Part model, mm, in its own coordinate system. Round coordinates to 2 decimals unless told otherwise and drop trailing zeros. Write each loop counter-clockwise with the first axis right and the second up, starting at its lowest first coordinate (ties: lowest second). Pieces come first, ordered by that corner, then holes.
```python
from build123d import *

# Parameters (mm, degrees)
ESQUISSE1_W             = 310
ESQUISSE1_H             = 380
BOSS_EXTRU_1_DEPTH      = 4
CONG_1_R                = 5
ESQUISSE3_R             = 10.5
ESQUISSE3_R_2           = 11
ESQUISSE3_R_3           = 2.5
ENL_V_MAT_EXTRU_1_DEPTH = 10


with BuildPart() as part:
    # Esquisse1 → Boss.-Extru.1 (new body)
    with BuildSketch(Plane.XY):
        with Locations((135.939300038, -172.787610619)):
            Rectangle(ESQUISSE1_W, ESQUISSE1_H)
    extrude(amount=BOSS_EXTRU_1_DEPTH)

    # Congé1
    cong_1_edges = [part.edges().sort_by_distance(p)[0] for p in [
        (-19.060699962, 17.212389381, 2),
        (290.939300038, 17.212389381, 2),
        (290.939300038, -362.787610619, 2),
        (-19.060699962, -362.787610619, 2),
    ]]
    fillet(cong_1_edges, radius=CONG_1_R)

    # Esquisse3 → Enlèv. mat.-Extru.1 (cut)
    with BuildSketch(Plane(origin=(0, 0, 0), x_dir=(-1, 0, 0), z_dir=(0, 0, -1))):
        with Locations((-205.939300038, -7.787610619)):
            Circle(ESQUISSE3_R)
        with Locations((-135.939300038, -21.787610619)):
            Circle(ESQUISSE3_R_2)
        with Locations((-65.939300038, -7.787610619)):
            Circle(ESQUISSE3_R)
        with Locations(Location((-217.253008537, 3.52609788, 0), (0, 0, 180))):
            Circle(ESQUISSE3_R_3)
        with Locations(Location((-194.625591539, 3.52609788, 0), (0, 0, 180))):
            Circle(ESQUISSE3_R_3)
        with Locations(Location((-194.625591539, -19.101319118, 0), (0, 0, 180))):
            Circle(ESQUISSE3_R_3)
        with Locations(Location((-217.253008537, -19.101319118, 0), (0, 0, 180))):
            Circle(ESQUISSE3_R_3)
        with Locations(Location((-77.253008537, 3.52609788, 0), (0, 0, 180))):
            Circle(ESQUISSE3_R_3)
        with Locations(Location((-54.625591539, 3.52609788, 0), (0, 0, 180))):
            Circle(ESQUISSE3_R_3)
        with Locations(Location((-54.625591539, -19.101319118, 0), (0, 0, 180))):
            Circle(ESQUISSE3_R_3)
        with Locations(Location((-77.253008537, -19.101319118, 0), (0, 0, 180))):
            Circle(ESQUISSE3_R_3)
        with Locations(Location((-119.939300038, -21.787610619, 0), (0, 0, 180))):
            Circle(ESQUISSE3_R_3)
        with Locations(Location((-124.625591539, -10.47390212, 0), (0, 0, 180))):
            Circle(ESQUISSE3_R_3)
        with Locations(Location((-124.625591539, -33.101319118, 0), (0, 0, 180))):
            Circle(ESQUISSE3_R_3)
        with Locations(Location((-147.253008537, -33.101319118, 0), (0, 0, 180))):
            Circle(ESQUISSE3_R_3)
        with Locations(Location((-151.939300038, -21.787610619, 0), (0, 0, 180))):
            Circle(ESQUISSE3_R_3)
        with Locations(Location((-147.253008537, -10.47390212, 0), (0, 0, 180))):
            Circle(ESQUISSE3_R_3)
        with Locations((13.060699962, -56.787610619)):
            Circle(ESQUISSE3_R_3)
        with Locations((13.060699962, -356.787610619)):
            Circle(ESQUISSE3_R_3)
        with Locations((-284.939300038, -356.787610619)):
            Circle(ESQUISSE3_R_3)
        with Locations((-284.939300038, -56.787610619)):
            Circle(ESQUISSE3_R_3)
    extrude(amount=-ENL_V_MAT_EXTRU_1_DEPTH, mode=Mode.SUBTRACT)


solid = part.part
```
Q1. Drop a flat-ended pin along its axis: pin 1 (3 mm diameter, centred on x = 77.25, y = -19.1, fed in from +Z). Give the stop position or say it passes through.
Values follow:
pin 1: passes through
Q2. Wall check: L1, parallel to Y at x = 65, z = 2.95; L2, parallel to X at y = -3.5, z = 3.55; L3, parallel to Y at x = 201.5, z = 1.25. Give the ranges that are in metal, low to high.
Values follow:
L1: y = -362.79 to -18.25, 2.67 to 17.21
L2: x = -19.06 to 56.35, 75.52 to 196.35, 215.52 to 290.94
L3: y = -362.79 to -17.3, 1.73 to 17.21
Q3. Mould opens along X. For faces 1 (the flat face through (134, -170, 0)), 2 (the cylindrical face through (55.924, -4.634, 1.972)) say: +X half, -X half, draft (parallel to the pull), parting line (faces both ways), or undercut.
Values follow:
face 1: draft
face 2: undercut
Q4. Cut at A-A on x = 133.5. Write the cut outline in (y, z), plus the area to 3 significant figures.
Values follow:
outline: (-362.79, 0) - (-32.51, 0) - (-32.51, 4) - (-362.79, 4) - close; (-11.06, 0) - (17.21, 0) - (17.21, 4) - (-11.06, 4) - close
area: 1,430 mm2
